Design review of the part built by this model. Coordinates are the model's own, in mm. A direction names the side the tool comes from. Give positions to 0.01 mm unless a question says otherwise; leave off trailing zeros. Order: outer loops, then holes, each group sorted by start corner. A loop starts at its lowest first (then second) coordinate and runs counter-clockwise, first axis right, second up. Notation, with made-up numbers: (-8, -30.75) -> (23, -30.75) arc R19 cw to (23, -26.75) -> close; hole circle Ø4 at (3.25, 11). An arc over 180 degrees is marked (long way). Return JSON: item names as keys, results as strings.
Autodesk Fusion 360 part; units mm, degrees
sketch "Sketch1" plane through (0, 0, 0) normal (0, 0, 1) x (1, 0, 0)
  line L0 (0, 0) -> (200, 0)
  line L1 (200, 0) -> (200, -100)
  line L2 (200, -100) -> (0, -100)
  line L3 (0, -100) -> (0, 0)
  dimension "d1" = 200
  dimension "d2" = 100
extrude "Extrude1" add sketch "Sketch1" along normal blind 40
sketch "Sketch2" plane through (0, 0, 40) normal (0, 0, 1) x (-1, 0, 0)
  line L0 (0, 100) -> (-200, 100)
  line L1 (-200, 100) -> (-200, 0)
  line L2 (-200, 0) -> (0, 0)
  line L3 (0, 0) -> (0, 100)
  line L4 (-200, 0) -> (-170, 0)
  line L5 (-170, 100) -> (-170, 0)
  line L6 (-200, 100) -> (-170, 100)
extrude "Extrude2" add sketch "Sketch2" along normal blind 40 contours L0 L1 L2 L4 L5 L6
sketch "Sketch3" plane through (170, 0, 0) normal (-1, 0, 0) x (0, -1, 0)
  line L0 (0, 40) -> (100, 40)
  line L1 (100, 40) -> (100, 80)
  line L2 (100, 80) -> (0, 80)
  line L3 (0, 80) -> (0, 40)
  arc A0 (90, 40) -> (10, 40) centre (50, 40) ccw
  dimension "d7" = 80
extrude "Extrude3" cut sketch "Sketch3" against normal blind 30 contours L0 L2 L3 A0 | L0 L1 L2 A0
sketch "Sketch4" plane through (0, 0, 0) normal (-1, 0, 0) x (0, -1, 0)
  line L0 (0, 0) -> (100, 0)
  line L1 (100, 0) -> (100, 40)
  line L2 (100, 40) -> (0, 40)
  line L3 (0, 40) -> (0, 0)
  line L4 (50, 30) -> (40, 30)
  line L5 (40, 30) -> (40, 15.5434)
  line L6 (40, 15.5434) -> (30, 15.5434)
  line L7 (30, 15.5434) -> (30, 0)
  line L8 (50, 30) -> (60, 30)
  line L9 (60, 30) -> (60, 16)
  line L10 (60, 16) -> (70, 16)
  line L11 (70, 16) -> (70, 0)
extrude "Extrude4" cut sketch "Sketch4" against normal blind 200 contours L0 L4 L5 L6 L7 L8 L9 L10 L11
sketch "Sketch5" plane through (0, 0, 40) normal (0, 0, 1) x (-1, 0, 0)
  line L0 (-170, 90) -> (-170, 10)
  line L1 (-170, 10) -> (-200, 10)
  line L2 (-200, 10) -> (-200, 0)
  line L3 (-200, 0) -> (0, 0)
  line L4 (0, 0) -> (0, 100)
  line L5 (0, 100) -> (-200, 100)
  line L6 (-200, 100) -> (-200, 90)
  line L7 (-200, 90) -> (-170, 90)
  line L8 (0, 0) -> (-70, 0)
  line L9 (-70, 0) -> (-70, 100)
  line L10 (-70, 100) -> (0, 100)
  line L11 (0, 100) -> (0, 0)
extrude "Extrude5" add sketch "Sketch5" along normal blind 55 contours L3 L4 L5 L8 L9 L10 L11
sketch "Sketch6" plane through (0, 0, 95) normal (0, 0, 1) x (-1, 0, 0)
  line L0 (0, 100) -> (-70, 100)
  line L1 (-70, 100) -> (-70, 0)
  line L2 (-70, 0) -> (0, 0)
  line L3 (0, 0) -> (0, 100)
  line L4 (0, 0) -> (-16.6169, 0)
  line L5 (-16.6169, 0) -> (-16.6169, 100)
  line L6 (-16.6169, 100) -> (0, 100)
  line L7 (0, 100) -> (0, 0)
extrude "Extrude6" cut sketch "Sketch6" against normal blind 55 contours L0 L2 L3 L4 L5 L6 L7
sketch "Sketch7" plane through (0, -100, 0) normal (0, -1, 0) x (1, 0, 0)
  line L0 (16.6169, 40) -> (0, 40)
  line L1 (0, 40) -> (0, 0)
  line L2 (0, 0) -> (200, 0)
  line L3 (200, 0) -> (200, 40)
  line L4 (200, 40) -> (70, 40)
  line L5 (70, 40) -> (70, 95)
  line L6 (70, 95) -> (16.6169, 95)
  line L7 (16.6169, 95) -> (16.6169, 40)
  arc A0 (70, 93.3831) -> (16.6169, 40) centre (70, 40) ccw
  line L8 (70, 93.3831) -> (16.6169, 93.3831)
extrude "Extrude7" cut sketch "Sketch7" against normal blind 200 contours L5 L6 L7 L8
sketch "Sketch8" plane through (0, -100, 0) normal (0, -1, 0) x (1, 0, 0)
  line L0 (70, 93.3831) -> (16.6169, 93.3831)
  line L1 (16.6169, 93.3831) -> (16.6169, 40)
  line L2 (16.6169, 40) -> (0, 40)
  line L3 (0, 40) -> (0, 0)
  line L4 (0, 0) -> (200, 0)
  line L5 (200, 0) -> (200, 40)
  line L6 (200, 40) -> (70, 40)
  line L7 (70, 40) -> (70, 93.3831)
  arc A0 (70, 93.3831) -> (16.6169, 40) centre (70, 40) ccw
extrude "Extrude8" cut sketch "Sketch8" against normal blind 200 contours L0 L1 A0
sketch "Sketch9" plane through (0, 0, 40) normal (0, 0, 1) x (-1, 0, 0)
  line L0 (-70, 0) -> (-70, 100)
  line L1 (-70, 100) -> (-200, 100)
  line L2 (-200, 100) -> (-200, 90)
  line L3 (-200, 90) -> (-170, 90)
  line L4 (-170, 90) -> (-170, 10)
  line L5 (-170, 10) -> (-200, 10)
  line L6 (-200, 10) -> (-200, 0)
  line L7 (-200, 0) -> (-70, 0)
  line L8 (-170, 0) -> (-170, 40)
  line L9 (-170, 40) -> (-70, 40)
  line L10 (-170, 100) -> (-170, 60)
  line L11 (-170, 60) -> (-70, 60)
  dimension "d20" = 40
  dimension "d21" = 40
extrude "Extrude9" cut sketch "Sketch9" against normal blind 10 contours L0 L4 L7 L8 L9 | L0 L1 L4 L10 L11
Item 1: Mouldability with a two-part tool opening along X and no side actions: class faces 1 (the face through (99, -70, 8)), 2 (the face through (121, -20, 30)), 3 (the face through (32.67, -50.7, 78.16)) as released by +X, released by -X, zero draft, split by the parting line, or undercut.
Result set:
{"face 1": "zero draft", "face 2": "undercut", "face 3": "released by -X"}
Item 2: Add section D-D (z = 72). Give the boundary of the cut face in (x, y), plus the area to 3 significant figures.
Result set:
{"outline": "(27.27, -100) -> (70, -100) -> (70, 0) -> (27.27, 0) -> close; (170, -74) -> (200, -74) -> (200, -26) -> (170, -26) -> close", "area": "5,710 mm^2"}
Item 3: Add section A-A (z = 13). Give the boundary of the cut face in (x, y).
Result set:
{"outline": "(0, -100) -> (200, -100) -> (200, -70) -> (0, -70) -> close; (0, -30) -> (200, -30) -> (200, 0) -> (0, 0) -> close"}
Item 4: Add section C-C (y = -50). Give the boundary of the cut face in (x, z).
Result set:
{"outline": "(0, 30) -> (200, 30) -> (200, 80) -> (170, 80) -> (170, 40) -> (70, 40) -> (70, 93.38) arc R53.38 ccw to (16.62, 40) -> (0, 40) -> close"}
Item 5: For pin 1 (22 mm diameter, centred on x = 114.5, y = -46, fed in from +Z); pin 2 (20 mm diameter, centred on x = 108.5, y = -83, fed in from +Z); pin 3 (8 mm diameter, centred on x = 151, y = -47, fed in from -Z), all flat-tipped, find the tip position at first contact; note any pin that passes through.
Result set:
{"pin 1": "stops at z = 40", "pin 2": "stops at z = 30", "pin 3": "stops at z = 30"}
Item 6: Wall thickness on L1, parallel to Y at x = 97, z = 6.5; L2, parallel to Y at x = 172.5, z = 21; L3, parallel to Z at x = 167.5, y = -76.5: over which ranges is each line inside the solid? List them lowest first. Write a range as [from, to].
Result set:
{"L1": "y = [-100, -70], [-30, 0]", "L2": "y = [-100, -60], [-40, 0]", "L3": "z = [0, 30]"}
Item 7: Machinability: for faces 4 (the face through (185, -5, 40)), 5 (the face through (185, -95, 40)), 6 (the face through (170, -51, 50)), which of the approach directions +Z, -Z, +X, -X, +Y, -Y give a long, thin tool a straight path to every point of the face, cutting with its end or side? Answer none if there is none.
Result set:
{"face 4": "+Z, +X, +Y", "face 5": "+Z, +X, -Y", "face 6": "+Z"}
